```python
from build123d import *

# Parameters (mm, degrees)
SKETCH_1_W          = 42
SKETCH_1_H          = 226
EXTRUDE_1_DEPTH     = 9.5
SKETCH_2_R          = 11.5
CUT_EXTRUDE_1_DEPTH = 231.065751471
SKETCH_3_W          = 16
SKETCH_3_H          = 9.5
EXTRUDE_2_DEPTH     = 9.5
SKETCH_4_R          = 4.4
CUT_EXTRUDE_2_DEPTH = 3
SKETCH_5_R          = 1.6
CUT_EXTRUDE_3_DEPTH = 231.065751471
SKETCH_6_R          = 2
CUT_EXTRUDE_6_DEPTH = 231.065751471
SKETCH_7_R          = 1.9
CUT_EXTRUDE_7_DEPTH = 231.065751471
SKETCH_9_R          = 4
CUT_EXTRUDE_8_DEPTH = 4


with BuildPart() as part:
    # 草图1 → 凸台-拉伸1 (new body)
    with BuildSketch(Plane(origin=(0, 0, 0), x_dir=(1, 0, 0), z_dir=(0, 1, 0))):
        with Locations((21, -113)):
            Rectangle(SKETCH_1_W, SKETCH_1_H)
    extrude(amount=EXTRUDE_1_DEPTH)

    # 草图2 → 切除-拉伸1 (cut, through all)
    with BuildSketch(Plane(origin=(0, 9.5, 0), x_dir=(1, 0, 0), z_dir=(0, 1, 0))):
        with Locations(Location((21, -113, 0), (0, 0, 270))):
            Circle(SKETCH_2_R)
    extrude(amount=-CUT_EXTRUDE_1_DEPTH, mode=Mode.SUBTRACT)

    # 草图3 → 凸台-拉伸2 (add)
    with BuildSketch(Plane.ZY):
        with Locations((8, 4.75)):
            Rectangle(SKETCH_3_W, SKETCH_3_H)
        with Locations((218, 4.75)):
            Rectangle(SKETCH_3_W, SKETCH_3_H)
    extrude(amount=EXTRUDE_2_DEPTH)

    # 草图4 → 切除-拉伸2 (cut)
    with BuildSketch(Plane(origin=(0, 9.5, 0), x_dir=(1, 0, 0), z_dir=(0, 1, 0))):
        with Locations(Location((20.47, -201.526194604, 0), (0, 0, 270))):
            Circle(SKETCH_4_R)
        with Locations(Location((20.47, -24.473805396, 0), (0, 0, 270))):
            Circle(SKETCH_4_R)
    extrude(amount=-CUT_EXTRUDE_2_DEPTH, mode=Mode.SUBTRACT)

    # 草图5 → 切除-拉伸3 (cut, through all)
    with BuildSketch(Plane.XZ):
        with Locations(Location((5.5, 97.5, 0), (0, 0, 270))):
            Circle(SKETCH_5_R)
        with Locations(Location((5.5, 128.5, 0), (0, 0, 270))):
            Circle(SKETCH_5_R)
        with Locations(Location((36.5, 97.5, 0), (0, 0, 270))):
            Circle(SKETCH_5_R)
        with Locations(Location((36.5, 128.5, 0), (0, 0, 270))):
            Circle(SKETCH_5_R)
    extrude(amount=-CUT_EXTRUDE_3_DEPTH, mode=Mode.SUBTRACT)

    # 草图6 → 切除-拉伸6 (cut, through all)
    with BuildSketch(Plane(origin=(0, 9.5, 0), x_dir=(1, 0, 0), z_dir=(0, 1, 0))):
        with Locations(Location((20.47, -201.526194604, 0), (0, 0, 270))):
            Circle(SKETCH_6_R)
        with Locations(Location((20.47, -24.473805396, 0), (0, 0, 270))):
            Circle(SKETCH_6_R)
    extrude(amount=-CUT_EXTRUDE_6_DEPTH, mode=Mode.SUBTRACT)

    # 草图7 → 切除-拉伸7 (cut, through all)
    with BuildSketch(Plane(origin=(0, 9.5, 0), x_dir=(1, 0, 0), z_dir=(0, 1, 0))):
        with Locations(Location((8, -220.8, 0), (0, 0, 270))):
            Circle(SKETCH_7_R)
        with Locations(Location((26.938917342, -220.8, 0), (0, 0, 270))):
            Circle(SKETCH_7_R)
    cut_extrude_7 = extrude(amount=-CUT_EXTRUDE_7_DEPTH, mode=Mode.SUBTRACT)

    # 草图9 → 切除-拉伸8 (cut)
    with BuildSketch(Plane(origin=(0, 9.5, 0), x_dir=(1, 0, 0), z_dir=(0, 1, 0))):
        with Locations(Location((8, -220.8, 0), (0, 0, 270))):
            Circle(SKETCH_9_R)
        with Locations(Location((26.938917342, -220.8, 0), (0, 0, 270))):
            Circle(SKETCH_9_R)
    cut_extrude_8 = extrude(amount=-CUT_EXTRUDE_8_DEPTH, mode=Mode.SUBTRACT)

    # 镜向1: 切除-拉伸7, 切除-拉伸8 across plane
    add(cut_extrude_7.mirror(Plane.XY.offset(113)), mode=Mode.SUBTRACT)
    add(cut_extrude_8.mirror(Plane.XY.offset(113)), mode=Mode.SUBTRACT)


solid = part.part
```
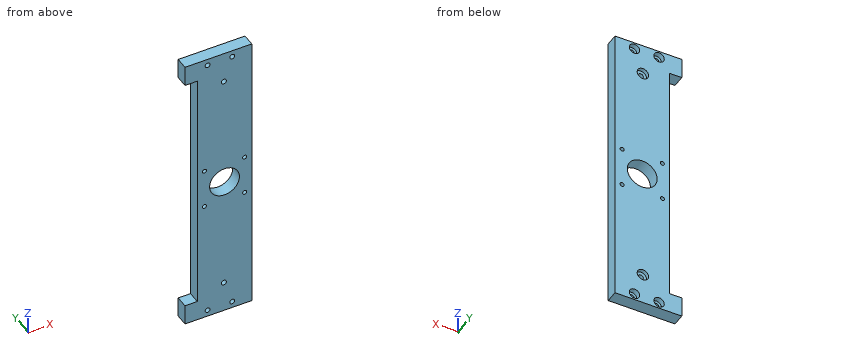
Design review of the part built by this model. Coordinates are the model's own, in mm. Give positions to 0.01 mm unless a question says otherwise; leave off trailing zeros. Loops run counter-clockwise (first coordinate to the right, second up) from the corner with the lowest first, then second, coordinate; pieces in that order, holes last. Notation, with made-up numbers: (7, 70) -> (36, 70) arc R33 cw to (36, 98) -> close; hole circle Ø5 at (-24, 20). An arc over 180 degrees is marked (long way). One line per item, written item: value.
Q1. We need section D-D on z = 113. Give the boundary of the cut face in (x, y).
Numbers:
outline: (0, 0) -> (9.5, 0) -> (9.5, 9.5) -> (0, 9.5) -> close; (32.5, 0) -> (42, 0) -> (42, 9.5) -> (32.5, 9.5) -> close
Q2. For pin 1 Ø1.9 at (x, z) = (5.5, 128.5) entering from -Y; pin 2 Ø2.5 at (x, z) = (7.5, 220) entering from +Y; pin 3 Ø3 at (y, z) = (4, 112.5) entering from -X, all flat-tipped, find the tip position at first contact; note any pin that passes through.
Numbers:
pin 1: passes through
pin 2: stops at y = 5.5
pin 3: stops at x = 0
Q3. We need section A-A on z = 220.8. Give the boundary of the cut face in (x, y).
Numbers:
outline: (-9.5, 0) -> (6.1, 0) -> (6.1, 5.5) -> (4, 5.5) -> (4, 9.5) -> (-9.5, 9.5) -> close; (9.9, 0) -> (25.04, 0) -> (25.04, 5.5) -> (22.94, 5.5) -> (22.94, 9.5) -> (12, 9.5) -> (12, 5.5) -> (9.9, 5.5) -> close; (28.84, 0) -> (42, 0) -> (42, 9.5) -> (30.94, 9.5) -> (30.94, 5.5) -> (28.84, 5.5) -> close
Q4. For L1, parallel to X at y = 4.2, z = 220.8; L2, parallel to Z at x = 20, y = 8; L3, parallel to X at y = 8.45, z = 220.8, list the stretches that pass through material, from the lowest coordinate up.
Numbers:
L1: x = -9.5 to 6.1, 9.9 to 25.04, 28.84 to 42
L2: z = 0 to 20.1, 28.85 to 101.54, 124.46 to 197.15, 205.9 to 226
L3: x = -9.5 to 4, 12 to 22.94, 30.94 to 42
Q5. We need section C-C on y = 2.75. Give the number of separate pieces and of enclosed holes in the cut face, and give its area (3 significant figures).
Numbers:
separate pieces: 1
enclosed holes: 11
area: 9,280 mm^2
Q6. We need section B-B on x = -2.5. Give the boundary of the cut face in (y, z), and give its area (3 significant figures).
Numbers:
outline: (0, 0) -> (9.5, 0) -> (9.5, 16) -> (0, 16) -> close; (0, 210) -> (9.5, 210) -> (9.5, 226) -> (0, 226) -> close
area: 304 mm^2
